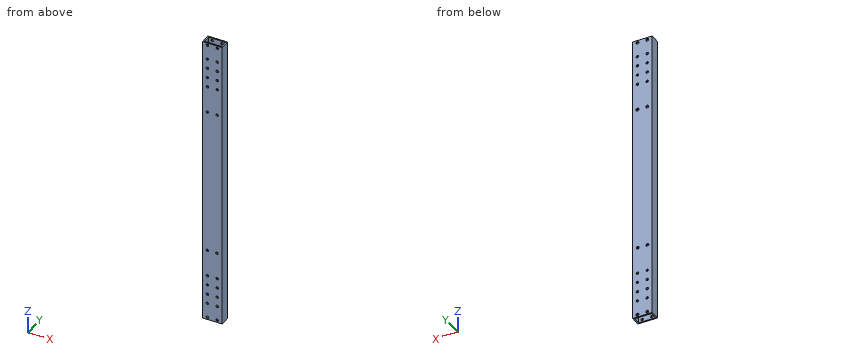
```python
from build123d import *

# Parameters (mm, degrees)
SKETCH1_W                             = 50.8
SKETCH1_H                             = 25.4
SKETCH1_W_2                           = 44.45
SKETCH1_H_2                           = 19.05
BOSS_EXTRUDE1_DEPTH                   = 762
F_1_4_0_25_DIAMETER_HOLE1_D           = 6.35
F_1_4_0_25_DIAMETER_HOLE1_CSINK_D     = 7.62
F_1_4_0_25_DIAMETER_HOLE1_CSINK_ANGLE = 90
F_1_4_0_25_DIAMETER_HOLE2_D           = 6.35
F_1_4_0_25_DIAMETER_HOLE2_CSINK_D     = 7.62
F_1_4_0_25_DIAMETER_HOLE2_CSINK_ANGLE = 90
CUT_EXTRUDE1_DEPTH                    = 765.11373499
CUT_EXTRUDE1_DEPTH_BACK               = 765.11373499
SKETCH9_R                             = 3.175


with BuildPart() as part:
    # Sketch1 → Boss-Extrude1 (new body)
    with BuildSketch(Plane.XY):
        with Locations((25.4, 12.7)):
            Rectangle(SKETCH1_W, SKETCH1_H)
        with Locations((25.4, 12.7)):
            Rectangle(SKETCH1_W_2, SKETCH1_H_2, mode=Mode.SUBTRACT)
    extrude(amount=BOSS_EXTRUDE1_DEPTH)

    # 1/4 (0.25) Diameter Hole1 (through all)
    with Locations(Plane(origin=(0, 25.4, 0), x_dir=(1, 0, 0), z_dir=(0, 1, 0))):
        with Locations((12.7, -6.35), (38.1, -6.35), (12.339930778, -190.5), (37.190506558, -190.5)):
            CounterSinkHole(F_1_4_0_25_DIAMETER_HOLE1_D / 2, F_1_4_0_25_DIAMETER_HOLE1_CSINK_D / 2, counter_sink_angle=F_1_4_0_25_DIAMETER_HOLE1_CSINK_ANGLE)

    # 1/4 (0.25) Diameter Hole2 (through all)
    with Locations(Plane(origin=(0, 25.4, 0), x_dir=(1, 0, 0), z_dir=(0, 1, 0))):
        with Locations((12.7, -755.65), (38.1, -755.65), (38.1, -571.5), (12.7, -571.5)):
            CounterSinkHole(F_1_4_0_25_DIAMETER_HOLE2_D / 2, F_1_4_0_25_DIAMETER_HOLE2_CSINK_D / 2, counter_sink_angle=F_1_4_0_25_DIAMETER_HOLE2_CSINK_ANGLE)

    # Sketch9 → Cut-Extrude1 (cut, two sides: drawn at the far end of the back side and taken through both)
    with BuildSketch(Plane(origin=(0, 25.4, 0), x_dir=(1, 0, 0), z_dir=(0, 1, 0)).offset(-CUT_EXTRUDE1_DEPTH_BACK)):
        with Locations(Location((12.7, -95.25, 0), (0, 0, 270))):
            Circle(SKETCH9_R)
        with Locations(Location((38.1, -95.25, 0), (0, 0, 270))):
            Circle(SKETCH9_R)
        with Locations(Location((12.7, -69.85, 0), (0, 0, 270))):
            Circle(SKETCH9_R)
        with Locations(Location((38.1, -69.85, 0), (0, 0, 270))):
            Circle(SKETCH9_R)
        with Locations(Location((12.7, -44.45, 0), (0, 0, 270))):
            Circle(SKETCH9_R)
        with Locations(Location((38.1, -44.45, 0), (0, 0, 270))):
            Circle(SKETCH9_R)
        with Locations(Location((38.1, -120.65, 0), (0, 0, 270))):
            Circle(SKETCH9_R)
        with Locations(Location((12.7, -120.65, 0), (0, 0, 270))):
            Circle(SKETCH9_R)
        with Locations(Location((12.7, -641.35, 0), (0, 0, 270))):
            Circle(SKETCH9_R)
        with Locations(Location((38.1, -641.35, 0), (0, 0, 270))):
            Circle(SKETCH9_R)
        with Locations(Location((38.1, -666.75, 0), (0, 0, 270))):
            Circle(SKETCH9_R)
        with Locations(Location((12.7, -666.75, 0), (0, 0, 270))):
            Circle(SKETCH9_R)
        with Locations(Location((12.7, -692.15, 0), (0, 0, 270))):
            Circle(SKETCH9_R)
        with Locations(Location((38.1, -692.15, 0), (0, 0, 270))):
            Circle(SKETCH9_R)
        with Locations(Location((38.1, -717.55, 0), (0, 0, 270))):
            Circle(SKETCH9_R)
        with Locations(Location((12.7, -717.55, 0), (0, 0, 270))):
            Circle(SKETCH9_R)
    extrude(amount=CUT_EXTRUDE1_DEPTH + CUT_EXTRUDE1_DEPTH_BACK, mode=Mode.SUBTRACT)


solid = part.part
```
The model under review builds one solid part; all positions refer to its coordinate system, in mm. Coordinates: 2 decimals unless noted, no trailing zeros. Write each loop counter-clockwise with the first axis right and the second up, starting at its lowest first coordinate (ties: lowest second). Pieces come first, ordered by that corner, then holes. Notation, with made-up numbers: (77, 24) - (103, 24) arc R19 ccw to (103, 45) - close; hole circle Ø10 at (48.5, -1.75). An arc over 180 degrees is marked (long way). Answer in a Markdown table with one row per item. Add a question column.
Q1. Consider section A-A on y = 14.5. Give the boundary of the cut face in (x, z) (3 decimals), then the cut area to 3 significant figures.
Q2. Clearance check with a flat-ended pin moving along its axis: pin 1 (5.5 mm diameter, centred on x = 12.7, z = 692.15, fed in from +Y). State where the tip first meets the part, or that it passes through.
Q3. Consider section C-C on x = 24. Give the boundary of the cut face in (y, z) (3 decimals), then the cut area to 3 significant figures.
Q4. To check wall thickness, follow line 1 along X through (y, z) = (23.8, 571.5) (3 decimals); line 2 along Y through (x, z) = (5, 50.5) (3 decimals); line 3 along X through (y, z) = (21.5, 517.5) (3 decimals). State the ranges of each line that lie inside material, in increasing order. Write a range as from..to.
Q5. Consider section B-B on z = 459.5. Give the boundary of the cut face in (x, y) (3 decimals).
Answers below:
| question | item | result |
|---|---|---|
| 1 | outline | (0, 0) - (3.175, 0) - (3.175, 762) - (0, 762) - close; (47.625, 0) - (50.8, 0) - (50.8, 762) - (47.625, 762) - close |
| 1 | area | 4,840 mm² |
| 2 | pin 1 | through |
| 3 | outline | (0, 0) - (3.175, 0) - (3.175, 762) - (0, 762) - close; (22.225, 0) - (25.4, 0) - (25.4, 762) - (22.225, 762) - close |
| 3 | area | 4,840 mm² |
| 4 | line 1 | 0..9.525, 15.875..34.925, 41.275..50.8 |
| 4 | line 2 | 0..3.175, 22.225..25.4 |
| 4 | line 3 | 0..3.175, 47.625..50.8 |
| 5 | outline | (0, 0) - (50.8, 0) - (50.8, 25.4) - (0, 25.4) - close; hole (3.175, 3.175) - (47.625, 3.175) - (47.625, 22.225) - (3.175, 22.225) - close |
